```python
from build123d import *

# Parameters (mm, degrees)
SKETCH1_W           = 70
SKETCH1_H           = 35
BOSS_EXTRUDE1_DEPTH = 10
FILLET1_R           = 4.5
SKETCH2_R           = 1.65
CUT_EXTRUDE1_DEPTH  = 10
SKETCH3_W           = 51
SKETCH3_H           = 30
CUT_EXTRUDE2_DEPTH  = 8
SKETCH4_W           = 6.75
SKETCH4_H           = 8
CUT_EXTRUDE3_DEPTH  = 11
SKETCH5_W           = 8.5
SKETCH5_H           = 16
CUT_EXTRUDE5_DEPTH  = 8
SKETCH6_W           = 9.5
SKETCH6_H           = 7.5
CUT_EXTRUDE6_DEPTH  = 4
FILLET2_R           = 0.75
FILLET3_R           = 5
FILLET4_R           = 7
FILLET5_R           = 5
FILLET6_R           = 2


with BuildPart() as part:
    # Sketch1 → Boss-Extrude1 (new body)
    with BuildSketch(Plane.XY):
        Rectangle(SKETCH1_W, SKETCH1_H)
    extrude(amount=BOSS_EXTRUDE1_DEPTH)

    # Fillet1
    fillet1_edges = [part.edges().sort_by_distance(p)[0] for p in [
        (35, -17.5, 5),
        (-35, -17.5, 5),
        (-35, 17.5, 5),
        (35, 17.5, 5),
    ]]
    fillet(fillet1_edges, radius=FILLET1_R)

    # Sketch2 → Cut-Extrude1 (cut)
    with BuildSketch(Plane.XY.offset(10)):
        with Locations((-30.5, 13)):
            Circle(SKETCH2_R)
        with Locations((30.5, 13)):
            Circle(SKETCH2_R)
        with Locations((30.5, -13)):
            Circle(SKETCH2_R)
        with Locations((-30.5, -13)):
            Circle(SKETCH2_R)
    extrude(amount=-CUT_EXTRUDE1_DEPTH, mode=Mode.SUBTRACT)

    # Sketch3 → Cut-Extrude2 (cut)
    with BuildSketch(Plane(origin=(0, 0, 0), x_dir=(-1, 0, 0), z_dir=(0, 0, -1))):
        Rectangle(SKETCH3_W, SKETCH3_H)
    extrude(amount=-CUT_EXTRUDE2_DEPTH, mode=Mode.SUBTRACT)

    # Sketch4 → Cut-Extrude3 (cut)
    with BuildSketch(Plane(origin=(0, 0, 0), x_dir=(-1, 0, 0), z_dir=(0, 0, -1))):
        with Locations((31.625, 0)):
            Rectangle(SKETCH4_W, SKETCH4_H)
    extrude(amount=-CUT_EXTRUDE3_DEPTH, mode=Mode.SUBTRACT)

    # Sketch5 → Cut-Extrude5 (cut)
    with BuildSketch(Plane(origin=(0, 0, 0), x_dir=(-1, 0, 0), z_dir=(0, 0, -1))):
        with Locations((29.75, 0)):
            Rectangle(SKETCH5_W, SKETCH5_H)
    extrude(amount=-CUT_EXTRUDE5_DEPTH, mode=Mode.SUBTRACT)

    # Sketch6 → Cut-Extrude6 (cut)
    with BuildSketch(Plane(origin=(0, 0, 0), x_dir=(-1, 0, 0), z_dir=(0, 0, -1))):
        with Locations((-30.25, 0)):
            Rectangle(SKETCH6_W, SKETCH6_H)
    extrude(amount=-CUT_EXTRUDE6_DEPTH, mode=Mode.SUBTRACT)

    # Fillet2
    fillet2_edges = [part.edges().sort_by_distance(p)[0] for p in [
        (30.25, 3.75, 4),
        (30.25, -3.75, 4),
        (30.25, -3.75, 0),
        (30.25, 3.75, 0),
    ]]
    fillet(fillet2_edges, radius=FILLET2_R)

    # Fillet3
    fillet3_edges = [part.edges().sort_by_distance(p)[0] for p in [
        (25.5, -15, 4),
        (25.5, 15, 4),
    ]]
    fillet(fillet3_edges, radius=FILLET3_R)

    # Fillet4
    fillet4_edges = [part.edges().sort_by_distance(p)[0] for p in [
        (-25.5, -8, 4),
        (-25.5, 8, 4),
    ]]
    fillet(fillet4_edges, radius=FILLET4_R - 0.0001)  # a hair under: the kernel refuses the full size

    # Fillet5
    fillet5_edges = [part.edges().sort_by_distance(p)[0] for p in [
        (-25.5, 15, 4),
        (-25.5, -15, 4),
    ]]
    fillet(fillet5_edges, radius=FILLET5_R)

    # Fillet6
    fillet6_edges = [part.edges().sort_by_distance(p)[0] for p in [
        (-34, -8, 4),
        (-34, 8, 4),
    ]]
    fillet(fillet6_edges, radius=FILLET6_R)


solid = part.part
```
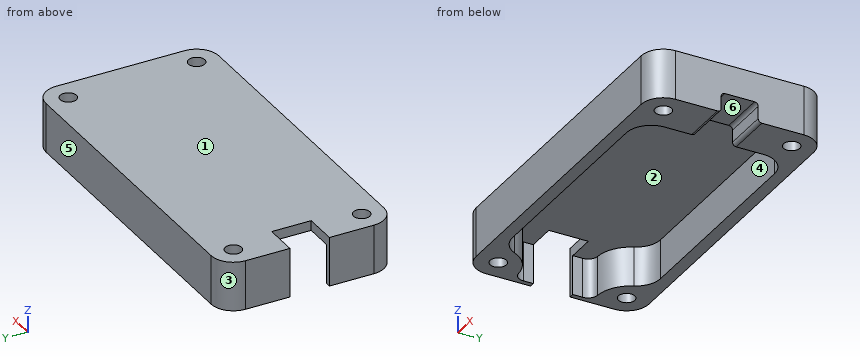
For this review, take the finished solid that the model builds, in its own axes (mm). Face numbers are marked on the shaded views. A direction names the side the tool comes from. Round coordinates to 2 decimals unless told otherwise and drop trailing zeros. Order: outer loops, then holes, each group sorted by start corner. A loop starts at its lowest first (then second) coordinate and runs counter-clockwise, first axis right, second up. Notation, with made-up numbers: (-16, 35.5) -> (26, 35.5) arc R17 cw to (26, 43.5) -> close; hole circle Ø7 at (57, 45.5). An arc over 180 degrees is marked (long way). Use a Markdown table: item, result.
Item 1: For line 1 along Y through (x, z) = (30.5, 3); line 2 along Y through (x, z) = (10, 4.75); line 3 along X through (y, z) = (5, 6), list the stretches that pass through material, from the lowest coordinate up. Write a range as [from, to].
Resolved:
| item | result |
|---|---|
| line 1 | y = [-17.5, -14.65], [-11.35, -3.75], [3.75, 11.35], [14.65, 17.5] |
| line 2 | y = [-17.5, -15], [15, 17.5] |
| line 3 | x = [-35, -34], [25.5, 35] |
Item 2: Take a section at B-B (z = 6.75). State how many separate pieces and enclosed holes the cut face has, plus the area to 3 significant figures.
Resolved:
| item | result |
|---|---|
| separate pieces | 1 |
| enclosed holes | 4 |
| area | 721 mm² |
Item 3: Draft analysis for pull direction X (two halves, no side actions). For the marked faces 1, 2 and 3, state which applies: +X half, -X half, draft (parallel to the pull), parting line (faces both ways), or undercut.
Resolved:
| item | result |
|---|---|
| face 1 | draft |
| face 2 | undercut |
| face 3 | -X half |
Item 4: Take a section at A-A (x = -10). State the section outline as (y, z) points, plus the area to 3 significant figures.
Resolved:
| item | result |
|---|---|
| outline | (-17.5, 0) -> (-15, 0) -> (-15, 8) -> (15, 8) -> (15, 0) -> (17.5, 0) -> (17.5, 10) -> (-17.5, 10) -> close |
| area | 110 mm² |
Item 5: Machinability: for the marked faces 4, 5 and 6, which of the approach directions +Z, -Z, +X, -X, +Y, -Y give a long, thin tool a straight path to every point of the face, cutting with its end or side? Answer none if there is none.
Resolved:
| item | result |
|---|---|
| face 4 | -Z |
| face 5 | +Z, -Z, +X, -X, +Y |
| face 6 | -Z, +X, -X |
Item 6: For pin 1 (6.5 mm diameter, centred on x = 28.5, y = 1, fed in from -Z); pin 2 (5 mm diameter, centred on y = 0.5, z = 7.5, fed in from -X), all flat-tipped, find the tip position at first contact; note any pin that passes through.
Resolved:
| item | result |
|---|---|
| pin 1 | stops at z = 0.04 |
| pin 2 | stops at x = -28.25 |
Item 7: Take a section at C-C (x = 23). State the section outline as (y, z) points, plus the area to 3 significant figures.
Resolved:
| item | result |
|---|---|
| outline | (-17.5, 0) -> (-14.33, 0) -> (-14.33, 8) -> (14.33, 8) -> (14.33, 0) -> (17.5, 0) -> (17.5, 10) -> (-17.5, 10) -> close |
| area | 121 mm² |
